Design review of the part built by this model. Coordinates are the model's own, in mm. Coordinates: 2 decimals unless noted, no trailing zeros. Use CSV: the item, a comma, the result in double quotes.
```python
from build123d import *

# Parameters (mm, degrees)
F0_W     = 59.4127969816
F0_H     = 115.0143891573
F1_DEPTH = 25.4
F2_R     = 5.08
F4_D     = 5.1054
F4_DEPTH = 16.51
F4_TIP   = 1.5338169022


with BuildPart() as f1:
    # F0 (on Top) → F1 (new body)
    with BuildSketch(Plane.XY):
        with Locations((-14.3670565449, 11.3745853305)):
            Rectangle(F0_W, F0_H)
    extrude(amount=F1_DEPTH)

    # F2
    f2_edges = [f1.edges().sort_by_distance(p)[0] for p in [
        (-44.073455, -46.132609, 12.7),
        (-14.367057, -46.132609, 25.4),
        (15.339342, -46.132609, 12.7),
        (-14.367057, -46.132609, 0),
    ]]
    fillet(f2_edges, radius=F2_R)

    # F4
    with Locations(Plane.XY.offset(25.4)):
        with Locations((-13.6958118528, 21.6659959406)):
            Hole(F4_D / 2, depth=F4_DEPTH)
            with Locations((0, 0, -(F4_DEPTH + F4_TIP / 2))):  # 118° drill point
                Cone(0, F4_D / 2, F4_TIP, mode=Mode.SUBTRACT)


solid = f1.part
```
Item 1: Draft analysis for pull direction Y (two halves, no side actions). For faces 1 (the face through (-15, 15, 25.4)), 2 (the face through (-14.87, 19.4, 17.03)), 3 (the face through (-13.951, -44.684, 23.872)), 4 (the face through (-13.491, 21.273, 7.623)), state which applies: pulls with the +Y half, pulls with the -Y half, needs draft (parallel to the pull), parting line crosses it, or undercut.
Checked values:
face 1,"needs draft"
face 2,"undercut"
face 3,"pulls with the -Y half"
face 4,"undercut"
Item 2: To check wall thickness, follow line 1 along Y through (x, z) = (-15, 14.25). State the ranges of the line that lie inside material, in increasing order.
Checked values:
line 1,"-46.13 to 19.47, 23.86 to 68.88"
Item 3: Clearance check with flat-ended pins moving along their axes: pin 1 (1 mm diameter, centred on x = -28, y = 4.5, fed in from -Z); pin 2 (3 mm diameter, centred on x = -13.7, y = 21.67, fed in from +Z). State where each tip first meets the part, or that it passes through.
Checked values:
pin 1,"z = 0"
pin 2,"z = 8.26"
